Here's how the part is built. I have some questions about the finished solid (model axes, mm). A direction names the side the tool comes from. Coordinates: 2 decimals unless noted, no trailing zeros. Write each loop counter-clockwise with the first axis right and the second up, starting at its lowest first coordinate (ties: lowest second). Pieces come first, ordered by that corner, then holes. Notation, with made-up numbers: (-23.5, 36.5) -> (0.5, 36.5) arc R13 ccw to (0.5, 59.5) -> close; hole circle Ø10 at (37, 63.25). An arc over 180 degrees is marked (long way). Put each result on its own line as item: value. Start each with the question number.
Item 1: I need wall thicknesses on line 1 (Y direction, x = -125, z = 0.8) (3 decimals); line 2 (Z direction, x = -90.5, y = 25); line 3 (X direction, y = -12, z = 3.5). Which ranges of each line are inside material? Lowest first, please. Write a range as [from, to].
Item 2: I want a section at C-C, the plane z = 1.5. List the corners of the cut face in (x, y) for me (3 decimals).
Item 3: I want a section at D-D, the plane y = 10. List the corners of the cut face in (x, z) for me.
Item 4: I want a section at A-A, the plane x = -61. List the corners of the cut face in (y, z) for me (3 decimals).
Item 5: I want a section at B-B, the plane y = -22.5. List the corners of the cut face in (x, z) for me.
Item 6: On a 3-axis mill with a long thin cutter (end or side, diameter ignored), from which of +Z, -Z, +X, -X, +Y, -Y can I reach the whole of each face in a straight line? I mean faces 1 (the face through (-97.3, 21.4, 5.5)), 2 (the face through (-141.92, 34.62, 2.86)), 3 (the face through (-34, -29, 4.35)), 4 (the face through (-79, 36.125, 3)), 5 (the face through (-74, -21.125, 3)). Say none if no direction works.
Item 7: For pin 1 (0.7 mm diameter, centred on y = 27, z = 5, fed in from +X); pin 2 (7.5 mm diameter, centred on x = -38, y = -32, fed in from +Z); pin 3 (1.6 mm diameter, centred on y = -10, z = 3.5, fed in from +X); pin 4 (3 mm diameter, centred on x = -136.98, y = -29.76, fed in from -Z), each with a flat end and sliding along its axis, tell me the tip position at first contact or that it passes through.
from build123d import *

# Parameters (mm, degrees)
F0_W         = 210
F0_H         = 52.25
F0_W_2       = 200
F0_H_2       = 42.25
F1_DEPTH     = 5.5
F0_W_3       = 230
F0_H_3       = 72.25
F2_DEPTH     = 5.65
F4_DEPTH     = 100
F5_R         = 5
F6_R         = 1.75
F7_DEPTH     = 25
F6_R_2       = 4
F8_DEPTH     = 3
F9_S6_R      = 1.75
F9_T7_DEPTH  = 7
F9_S13_R     = 1.75
F9_T14_DEPTH = 7


# Not quite as in the source:
# - a fillet or chamfer that OpenCascade refuses, or shapes differently, is made with other operations: its cross-section is extruded or revolved along the edge and cut away or added


with BuildPart() as f1:
    # F0 (on Top) → F1 (new body)
    with BuildSketch(Plane.XY):
        with Locations((-28.3456140757, 0)):
            Rectangle(F0_W, F0_H)
        with Locations((-28.3456140757, 0)):
            Rectangle(F0_W_2, F0_H_2, mode=Mode.SUBTRACT)
    extrude(amount=F1_DEPTH)

    # F0 (on Top) → F2 (join)
    with BuildSketch(Plane.XY):
        with Locations((-28.3456140757, 0)):
            Rectangle(F0_W_3, F0_H_3)
        with Locations((-28.3456140757, 0)):
            Rectangle(F0_W, F0_H, mode=Mode.SUBTRACT)
    extrude(amount=F2_DEPTH)

    # F3 (on face) → F4 (cut)
    with BuildSketch(Plane.XZ.offset(36.125)):
        Polygon((-48.3456140757, 5.65), (-48.3456140757, 4.35), (-18.3456140757, 4.35), (-18.3456140757, 0), (86.6543859243, 0), (86.6543859243, 5.65), align=None)
    extrude(amount=-F4_DEPTH, mode=Mode.SUBTRACT)

    # F5
    f5_edges = [f1.edges().sort_by_distance(p)[0] for p in [
        (-143.345614, 36.125, 2.825),
        (-143.345614, -36.125, 2.825),
    ]]
    fillet(f5_edges, radius=F5_R)

    # F6 (on face) → F7 (cut)
    with BuildSketch(Plane.XY):
        with Locations((-136.9816213846, 29.760915786)):
            Circle(F6_R)
        with Locations((-136.9816213846, -29.760915786)):
            Circle(F6_R)
    extrude(amount=F7_DEPTH, mode=Mode.SUBTRACT)

    # F6 (on face) → F8 (cut)
    with BuildSketch(Plane.XY):
        with Locations((-136.9816213846, -29.760915786)):
            Circle(F6_R_2)
        with Locations((-136.9816213846, -29.760915786)):
            Circle(F6_R, mode=Mode.SUBTRACT)
        with Locations((-136.9816213846, 29.760915786)):
            Circle(F6_R_2)
        with Locations((-136.9816213846, 29.760915786)):
            Circle(F6_R, mode=Mode.SUBTRACT)
    extrude(amount=F8_DEPTH, mode=Mode.SUBTRACT)

    # F9: chamfer of 3 x 2.2606621503 on 2 edges, made by hand


with BuildPart() as f9_tool2:
    # F9_s3 → F9_t4 (revolve)
    with BuildSketch(Plane.XZ.offset(-29.760915786)):
        Polygon((-132.9816213846, 0), (-135.2422835349, 3), (-132.9816213846, 3), align=None)
    revolve(axis=Axis((-136.9816213846, 29.760915786, 3), (0, 0, 1)))

    split(bisect_by=Plane.XY, keep=Keep.TOP)

    # F9_s6 → F9_t7 (cut, symmetric)
    with BuildSketch(Plane.XY.offset(1.5)):
        with Locations((-136.9816213846, 29.760915786)):
            Circle(F9_S6_R)
    extrude(amount=F9_T7_DEPTH, both=True, mode=Mode.SUBTRACT)


with BuildPart() as f1_1:
    add(f1.part)

    # F9_t1: union F9_tool2
    add(f9_tool2.part)


with BuildPart() as f9_tool9:
    # F9_s10 → F9_t11 (revolve)
    with BuildSketch(Plane.XZ.offset(29.760915786)):
        Polygon((-132.9816213846, 0), (-135.2422835349, 3), (-132.9816213846, 3), align=None)
    revolve(axis=Axis((-136.9816213846, -29.760915786, 3), (0, 0, 1)))

    split(bisect_by=Plane.XY, keep=Keep.TOP)

    # F9_s13 → F9_t14 (cut, symmetric)
    with BuildSketch(Plane.XY.offset(1.5)):
        with Locations((-136.9816213846, -29.760915786)):
            Circle(F9_S13_R)
    extrude(amount=F9_T14_DEPTH, both=True, mode=Mode.SUBTRACT)


with BuildPart() as f1_2:
    add(f1_1.part)

    # F9_t8: union F9_tool9
    add(f9_tool9.part)


solid = f1_2.part
Calculated:
1. line 1: y = [-36.125, -21.125], [21.125, 36.125]
1. line 2: z = [0, 5.5]
1. line 3: x = [-143.35, -128.35]
2. outline: (-143.346, -31.125) arc R5 ccw to (-138.346, -36.125) -> (-18.346, -36.125) -> (-18.346, -21.125) -> (-128.346, -21.125) -> (-128.346, 21.125) -> (-18.346, 21.125) -> (-18.346, 36.125) -> (-138.346, 36.125) arc R5 ccw to (-143.346, 31.125) -> close; hole circle Ø5.739 at (-136.982, -29.761); hole circle Ø5.739 at (-136.982, 29.761)
3. outline: (-143.35, 0) -> (-128.35, 0) -> (-128.35, 5.5) -> (-133.35, 5.5) -> (-133.35, 5.65) -> (-143.35, 5.65) -> close
4. outline: (-36.125, 0) -> (-21.125, 0) -> (-21.125, 5.5) -> (-26.125, 5.5) -> (-26.125, 5.65) -> (-36.125, 5.65) -> close; (21.125, 0) -> (36.125, 0) -> (36.125, 5.65) -> (26.125, 5.65) -> (26.125, 5.5) -> (21.125, 5.5) -> close
5. outline: (-143.35, 0) -> (-18.35, 0) -> (-18.35, 4.35) -> (-48.35, 4.35) -> (-48.35, 5.5) -> (-133.35, 5.5) -> (-133.35, 5.65) -> (-143.35, 5.65) -> close
6. face 1: +Z, +X
6. face 2: +Z, -Z, -X, +Y
6. face 3: +Z, +X, +Y, -Y
6. face 4: +Z, -Z, +X, -X, +Y
6. face 5: +Z, -Z, +X
7. pin 1: stops at x = -48.35
7. pin 2: stops at z = 4.35
7. pin 3: stops at x = -128.35
7. pin 4: passes through
